The model under review builds one solid part; all positions refer to its coordinate system, in mm. Coordinates: 2 decimals unless noted, no trailing zeros. One line per item, written item: value.
```python
from build123d import *

# Parameters (mm, degrees)
SKETCH1_R           = 3
SKETCH1_R_2         = 3.5
BOSS_EXTRUDE1_DEPTH = 9.525


with BuildPart() as part:
    # Sketch1 → Boss-Extrude1 (new body)
    with BuildSketch(Plane.XY):
        Polygon((-27.364320758, 113.012415756), (72.635679242, 113.012415756), (72.635679242, 7.787512308), (72.635679242, -131.987584244), (72.635679242, -186.987584244), (-27.364320758, -186.987584244), (-27.364320758, -131.987584244), (-27.364320758, 7.787512308), align=None)
        with Locations(Location((-12.364320758, 108.012415756, 0), (0, 0, 180))):
            Circle(SKETCH1_R, mode=Mode.SUBTRACT)
        with Locations(Location((57.635679242, 49.012415756, 0), (0, 0, 180))):
            Circle(SKETCH1_R, mode=Mode.SUBTRACT)
        with Locations(Location((-12.364320758, 49.012415756, 0), (0, 0, 180))):
            Circle(SKETCH1_R, mode=Mode.SUBTRACT)
        with Locations(Location((57.635679242, 108.012415756, 0), (0, 0, 180))):
            Circle(SKETCH1_R, mode=Mode.SUBTRACT)
        with Locations(Location((-12.364320758, -166.987584244, 0), (0, 0, 180))):
            Circle(SKETCH1_R_2, mode=Mode.SUBTRACT)
        with Locations(Location((57.635679242, -166.987584244, 0), (0, 0, 180))):
            Circle(SKETCH1_R_2, mode=Mode.SUBTRACT)
    extrude(amount=BOSS_EXTRUDE1_DEPTH)


solid = part.part
```
(1) Insertion check: pin 1 Ø3.5 at (x, y) = (57.64, 49.01) entering from -Z; pin 2 Ø5 at (x, y) = (33.5, -17.5) entering from -Z. Each pin has a flat end and moves straight along its axis. Give the tip position at first contact, or say it passes through.
Checks:
pin 1: through
pin 2: z = 0
(2) Draft analysis for pull direction Y (two halves, no side actions). For faces 1 (the face through (-11.61, -163.57, 4.7)), 2 (the face through (23, -186.988, 5)), 3 (the face through (22, 113.012, 5)), 4 (the face through (-27.364, -35, 5)), state which applies: pulls with the +Y half, pulls with the -Y half, needs draft (parallel to the pull), parting line crosses it, or undercut.
Checks:
face 1: undercut
face 2: pulls with the -Y half
face 3: pulls with the +Y half
face 4: needs draft
(3) To check wall thickness, follow L1, parallel to X at y = 47, z = 1.5; L2, parallel to Y at x = -11.5, z = 2. State the ranges of each line that lie inside material, in increasing order. Write a range as [from, to].
Checks:
L1: [-27.36, -14.59], [-10.14, 55.41], [59.86, 72.64]
L2: [-186.99, -170.38], [-163.6, 46.14], [51.89, 105.14], [110.89, 113.01]
